Here's how the part is built. I have some questions about the finished solid (model axes, mm). A direction names the side the tool comes from. Coordinates: 2 decimals unless noted, no trailing zeros. Write each loop counter-clockwise with the first axis right and the second up, starting at its lowest first coordinate (ties: lowest second). Pieces come first, ordered by that corner, then holes.
(1) Imagine slicing it at A-A, the plane z = 32. List the corners of the cut face in (x, y) for me, plus the area to 3 significant figures.
(2) Please list where these lines run through material, in increasing order: probe 1 along Z at (x, y) = (3.4, 9); probe 2 along Y at (x, z) = (0.8, 88.5); probe 3 along Z at (x, y) = (1.65, 83).
(3) Thinking about a two-plate mould opening in Z: for faces 1 (the flat face through (2, 94, 160)), 2 (the flat face through (2, 98, 140)), 3 (the flat face through (2, 96, 135)), 4 (the flat face through (2, 0, 150)), which applies, released by +Z, released by -Z, zero draft, split by the parting line, or undercut?
(4) Which directions (+Z, -Z, +X, -X, +Y, -Y) give clear straight access to the entire face, cutting with the end or side of a thin tool? Please do faces 5 (the flat face through (2, 92, 158)), 6 (the flat face through (2, 96, 95)), 7 (the flat face through (2, 80, 2)), 8 (the flat face through (2, 100, 25)).
(5) Imagine slicing it at B-B, the plane y = 26. List the corners of the cut face in (x, z) for me.
(6) For pin 1 Ø1.2 at (x, y) = (1.5, 3) entering from -Z; pin 2 Ø2 at (x, y) = (1, 99) entering from +Z; pin 3 Ø1.2 at (x, z) = (2.5, 137) entering from +Y; pin 4 Ø2 at (x, y) = (1.5, 97.5) entering from -Z, each with a flat end and sliding along its axis, tell me the tip position at first contact or that it passes through.
```python
from build123d import *

# Parameters (mm, degrees)
F0_W     = 100
F0_H     = 160
F1_DEPTH = 4
F2_W     = 4
F2_H     = 10
F3_DEPTH = 4
F4_W     = 4
F4_H     = 5
F4_W_2   = 88
F4_H_2   = 4
F5_DEPTH = 4
F7_DEPTH = 4


with BuildPart() as f1:
    # F0 (on Right) → F1 (new body)
    with BuildSketch(Plane.YZ):
        with Locations((50, 80)):
            Rectangle(F0_W, F0_H)
    extrude(amount=F1_DEPTH)

    # F2 (on face) → F3 (cut, through all)
    with BuildSketch(Plane.YZ.offset(4)):
        with Locations((98, 155)):
            Rectangle(F2_W, F2_H)
        with Locations((98, 135)):
            Rectangle(F2_W, F2_H)
        with Locations((98, 115)):
            Rectangle(F2_W, F2_H)
        with Locations((98, 95)):
            Rectangle(F2_W, F2_H)
        with Locations((98, 75)):
            Rectangle(F2_W, F2_H)
        with Locations((98, 55)):
            Rectangle(F2_W, F2_H)
        with Locations((98, 35)):
            Rectangle(F2_W, F2_H)
        with Locations((98, 15)):
            Rectangle(F2_W, F2_H)
    extrude(amount=-F3_DEPTH, mode=Mode.SUBTRACT)

    # F4 (on face) → F5 (cut, through all)
    with BuildSketch(Plane.YZ.offset(4)):
        with Locations((78, 2.5)):
            Rectangle(F4_W, F4_H)
        with Locations((48, 158)):
            Rectangle(F4_W_2, F4_H_2)
    extrude(amount=-F5_DEPTH, mode=Mode.SUBTRACT)

    # F6 (on face) → F7 (cut, through all)
    with BuildSketch(Plane.YZ.offset(4)):
        with BuildLine():
            Line((10, 140), (0, 140))
            Line((0, 140), (0, 0))
            Line((0, 0), (40, 0))
            Line((40, 0), (40, 10))
            Line((40, 10), (40, 40))
            Line((40, 40), (20, 80))
            Line((20, 80), (20, 130))
            ThreePointArc((20, 130), (17.071068, 137.071068), (10, 140))
        make_face()
        with BuildLine():
            Line((40, 10), (40, 0))
            Line((40, 0), (50, 0))
            ThreePointArc((50, 0), (42.928932, 2.928932), (40, 10))
        make_face()
    extrude(amount=-F7_DEPTH, mode=Mode.SUBTRACT)


solid = f1.part
```
Recorded:
1. outline: (0, 40) - (4, 40) - (4, 96) - (0, 96) - close
1. area: 224 mm2
2. probe 1: z = 140 to 156
2. probe 2: y = 20 to 100
2. probe 3: z = 0 to 156
3. face 1: released by +Z
3. face 2: undercut
3. face 3: undercut
3. face 4: zero draft
4. face 5: +Z, +X, -X
4. face 6: +X, -X, +Y
4. face 7: -Z, +X, -X
4. face 8: +Z, -Z, +X, -X, +Y
5. outline: (0, 68) - (4, 68) - (4, 156) - (0, 156) - close
6. pin 1: stops at z = 140
6. pin 2: stops at z = 150
6. pin 3: stops at y = 96
6. pin 4: stops at z = 0
